Geometry check sheet. Reference: the model listing, model coordinates, mm. A direction names the side the tool comes from. Coordinates: 2 decimals unless noted, no trailing zeros. Write each loop counter-clockwise with the first axis right and the second up, starting at its lowest first coordinate (ties: lowest second). Pieces come first, ordered by that corner, then holes. Notation, with made-up numbers: M -8.5,70 L 33.5,70 A13 ccw 33.5,85 Z; hole C -23.5,2 d10. An arc over 180 degrees is marked long. Answer as a JSON object with one key per item and string values. Group by question number.
```python
from build123d import *

# Parameters (mm, degrees)
SKETCH_1_W               = 800
SKETCH_1_H               = 2000
EXTRUDE_1_DEPTH          = 50
SKETCH_2_W               = 20
SKETCH_2_H               = 100
EXTRUDE_2_DEPTH          = 50
SKETCH_3_R               = 20
EXTRUDE_3_DEPTH          = 100
PATTERN_LINEAR_1_COUNT   = 2
PATTERN_LINEAR_1_PITCH   = 1200
SKETCH_4_R               = 30
EXTRUDE_4_DEPTH          = 10
SKETCH_5_R               = 10
EXTRUDE_5_DEPTH          = 40
EXTRUDE_6_DEPTH          = 20
FILLET_1_R               = 10
MIRROR_START             = 610
MIRROR_1_DEPTH           = 120
MIRROR_2_COPY_1_SKETCH_W = 20
MIRROR_2_COPY_1_SKETCH_H = 100
MIRROR_2_COPY_1_DEPTH    = 50
MIRROR_2_COPY_2_SKETCH_R = 20
MIRROR_2_COPY_2_DEPTH    = 100
DELETE_START             = 405
DELETE_FACE_1_DEPTH      = 1300


with BuildPart() as part:
    # Эскиз1 → Бобышка-Вытянуть1 (new body)
    with BuildSketch(Plane(origin=(46095.73955041, 0, 0), x_dir=(-1, 0, 0), z_dir=(0, 0, -1))):
        with Locations((45695.73955041, 1000)):
            Rectangle(SKETCH_1_W, SKETCH_1_H)
    extrude(amount=-EXTRUDE_1_DEPTH)

    # Эскиз2 → Бобышка-Вытянуть2 (add)
    with BuildSketch(Plane(origin=(0, 0, 0), x_dir=(-1, 0, 0), z_dir=(0, 0, -1))):
        with Locations((-10, 1655)):
            Rectangle(SKETCH_2_W, SKETCH_2_H)
    extrude_2 = extrude(amount=EXTRUDE_2_DEPTH)

    # Эскиз3 → Бобышка-Вытянуть3 (add)
    with BuildSketch(Plane(origin=(0, 1605, 0), x_dir=(-1, 0, 0), z_dir=(0, -1, 0))):
        with Locations((5, 30)):
            Circle(SKETCH_3_R)
    extrude_3 = extrude(amount=-EXTRUDE_3_DEPTH)

    # Линейный массив1: Бобышка-Вытянуть2, Бобышка-Вытянуть3 ×2
    with Locations(*[(0, -i * PATTERN_LINEAR_1_PITCH, 0) for i in range(1, PATTERN_LINEAR_1_COUNT)]):
        add(extrude_2)
        add(extrude_3)

    # Эскиз4 → Бобышка-Вытянуть4 (add)
    with BuildSketch(Plane(origin=(0, 0, 0), x_dir=(-1, 0, 0), z_dir=(0, 0, -1))):
        with Locations((-730, 1000)):
            Circle(SKETCH_4_R)
    extrude(amount=EXTRUDE_4_DEPTH)

    # Эскиз5 → Бобышка-Вытянуть5 (add)
    with BuildSketch(Plane(origin=(0, 0, -10), x_dir=(-1, 0, 0), z_dir=(0, 0, -1))):
        with Locations((-730, 1000)):
            Circle(SKETCH_5_R)
    extrude(amount=EXTRUDE_5_DEPTH)

    # Эскиз6 → Бобышка-Вытянуть6 (add)
    with BuildSketch(Plane(origin=(0, 0, -50), x_dir=(-1, 0, 0), z_dir=(0, 0, -1))):
        with BuildLine():
            Line((-730, 1010), (-610, 1010))
            ThreePointArc((-610, 1010), (-600, 1000), (-610, 990))
            Line((-610, 990), (-730, 990))
            ThreePointArc((-730, 990), (-740, 1000), (-730, 1010))
        make_face()
    extrude(amount=EXTRUDE_6_DEPTH)

    # Скругление1
    # the kernel refuses this fillet: 10 mm, written as the material it takes off along each edge
    with BuildSketch(Plane(origin=(755, 1010, -50), x_dir=(0, -1, 0), z_dir=(-1, 0, 0))) as fillet_1_piece_1_section:
        with BuildLine():
            CenterArc((FILLET_1_R, -FILLET_1_R), FILLET_1_R, 90, 90)
            Line((0, -FILLET_1_R), (0, 0))
            Line((0, 0), (FILLET_1_R, 0))
        make_face()
    fillet_1_piece_1 = extrude(amount=145, mode=Mode.PRIVATE)
    fillet_1_piece_1 = fillet_1_piece_1 - Plane(origin=(730, 1000, -50), x_dir=(-1, 0, 0), z_dir=(0, 0, 1)) * Cylinder(10, 330, mode=Mode.PRIVATE)
    add(fillet_1_piece_1, mode=Mode.SUBTRACT)
    with BuildSketch(Plane(origin=(610, 1000, -50), x_dir=(0, 1, 0), z_dir=(1, 0, 0))) as fillet_1_piece_2:
        with BuildLine():
            CenterArc((10 - FILLET_1_R, -FILLET_1_R), FILLET_1_R, 0, 90)
            Line((10, -FILLET_1_R), (10, 0))
            Line((10, 0), (10 - FILLET_1_R, 0))
        make_face()
    revolve(axis=Axis((610, 1000, -50), (0, 0, 1)), revolution_arc=180, mode=Mode.SUBTRACT)
    with BuildSketch(Plane(origin=(730, 1010, -70), x_dir=(0, 0, 1), z_dir=(-1, 0, 0)), Plane(origin=(610, 990, -70), x_dir=(0, 0, 1), z_dir=(1, 0, 0))) as fillet_1_piece_3:
        with BuildLine():
            CenterArc((FILLET_1_R, -FILLET_1_R), FILLET_1_R, 90, 90)
            Line((0, -FILLET_1_R), (0, 0))
            Line((0, 0), (FILLET_1_R, 0))
        make_face()
    extrude(amount=120, mode=Mode.SUBTRACT)
    with BuildSketch(Plane(origin=(610, 1000, -70), x_dir=(0, 1, 0), z_dir=(1, 0, 0))) as fillet_1_piece_4:
        with BuildLine():
            CenterArc((10 - FILLET_1_R, FILLET_1_R), FILLET_1_R, 270, 90)
            Line((10 - FILLET_1_R, 0), (10, 0))
            Line((10, 0), (10, FILLET_1_R))
        make_face()
    revolve(axis=Axis((610, 1000, -70), (0, 0, 1)), revolution_arc=180, mode=Mode.SUBTRACT)
    with BuildSketch(Plane(origin=(730, 1000, -70), x_dir=(0, -1, 0), z_dir=(-1, 0, 0))) as fillet_1_piece_5:
        with BuildLine():
            CenterArc((10 - FILLET_1_R, FILLET_1_R), FILLET_1_R, 270, 90)
            Line((10 - FILLET_1_R, 0), (10, 0))
            Line((10, 0), (10, FILLET_1_R))
        make_face()
    revolve(axis=Axis((730, 1000, -70), (0, 0, 1)), revolution_arc=180, mode=Mode.SUBTRACT)
    with BuildSketch(Plane(origin=(730, 1000, -10), x_dir=(-1, 0, 0), z_dir=(0, -1, 0))) as fillet_1_piece_6:
        with BuildLine():
            CenterArc((30 - FILLET_1_R, -FILLET_1_R), FILLET_1_R, 0, 90)
            Line((30 - FILLET_1_R, 0), (30, 0))
            Line((30, 0), (30, -FILLET_1_R))
        make_face()
    revolve(axis=Axis((730, 1000, -10), (0, 0, -1)), mode=Mode.SUBTRACT)
    with BuildSketch(Plane(origin=(610, 990, -50), x_dir=(0, 1, 0), z_dir=(1, 0, 0))) as fillet_1_piece_7_section:
        with BuildLine():
            CenterArc((FILLET_1_R, -FILLET_1_R), FILLET_1_R, 90, 90)
            Line((0, -FILLET_1_R), (0, 0))
            Line((0, 0), (FILLET_1_R, 0))
        make_face()
    fillet_1_piece_7 = extrude(amount=145, mode=Mode.PRIVATE)
    fillet_1_piece_7 = fillet_1_piece_7 - Plane(origin=(730, 1000, -50), x_dir=(-1, 0, 0), z_dir=(0, 0, 1)) * Cylinder(10, 330, mode=Mode.PRIVATE)
    add(fillet_1_piece_7, mode=Mode.SUBTRACT)



with BuildPart() as body_2:
    # Зеркальное отражение1: read off the stored shape, not the designer's step
    # Зеркальное отражение1 outline → Зеркальное отражение1 (new body)
    with BuildSketch(Plane.YZ.offset(MIRROR_START)):
        with BuildLine():
            ThreePointArc((1000, 120), (992.928932188, 117.071067812), (990, 110))
            ThreePointArc((990, 110), (992.928932188, 102.928932188), (1000, 100))
            ThreePointArc((1000, 100), (1007.071067812, 102.928932188), (1010, 110))
            ThreePointArc((1010, 110), (1007.071067812, 117.071067812), (1000, 120))
        make_face()
    extrude(amount=MIRROR_1_DEPTH)


with BuildPart() as part_1:
    add(part.part)

    add(body_2.part)  # Mirror 1 2 merges body 2
    # Mirror 1 2 outline → Mirror 1 2 (revolve)
    with BuildSketch(Plane(origin=(730, 1000, 0), x_dir=(1, 0, 0), z_dir=(0, -1, 0))):
        with BuildLine():
            Line((10, 60), (10, 110))
            ThreePointArc((10, 110), (7.071067812, 117.071067812), (0, 120))
            Line((0, 120), (0, 50))
            Line((0, 50), (30, 50))
            ThreePointArc((30, 50), (27.071067812, 57.071067812), (20, 60))
            Line((20, 60), (10, 60))
        make_face()
    revolve(axis=Axis((730, 1000, 0), (0, 0, 1)))

    # Mirror 1 3 outline → Mirror 1 3 (revolve)
    with BuildSketch(Plane(origin=(0, 1000, 110), x_dir=(0, 1, 0), z_dir=(0, 0, -1))):
        with BuildLine():
            Line((0, 610), (0, 600))
            ThreePointArc((0, 600), (7.071067812, 602.928932188), (10, 610))
            Line((10, 610), (0, 610))
        make_face()
    revolve(axis=Axis((0, 1000, 110), (1, 0, 0)))

    # Зеркальное отражение2: Бобышка-Вытянуть2, Бобышка-Вытянуть3 across plane
    add(extrude_2.mirror(Plane(origin=(0, 0, 25), x_dir=(1, 0, 0), z_dir=(0, 0, -1))))
    add(extrude_3.mirror(Plane(origin=(0, 0, 25), x_dir=(1, 0, 0), z_dir=(0, 0, -1))))

    # Зеркальное отражение2 copy 1 sketch → Зеркальное отражение2 copy 1 (add)
    with BuildSketch(Plane(origin=(0, -1200, 50), x_dir=(-1, 0, 0), z_dir=(0, 0, 1))):
        with Locations((-10, -1655)):
            Rectangle(MIRROR_2_COPY_1_SKETCH_W, MIRROR_2_COPY_1_SKETCH_H)
    extrude(amount=MIRROR_2_COPY_1_DEPTH)

    # Зеркальное отражение2 copy 2 sketch → Зеркальное отражение2 copy 2 (add)
    with BuildSketch(Plane(origin=(0, 405, 50), x_dir=(-1, 0, 0), z_dir=(0, -1, 0))):
        with Locations((5, -30)):
            Circle(MIRROR_2_COPY_2_SKETCH_R)
    extrude(amount=-MIRROR_2_COPY_2_DEPTH)

    # Delete Face 1: read off the stored shape, not the designer's step
    # Delete Face 1 outline → Delete Face 1 (cut)
    with BuildSketch(Plane(origin=(0, 0, 0), x_dir=(1, 0, 0), z_dir=(0, 1, 0)).offset(DELETE_START)):
        with BuildLine():
            Line((20, 50), (0, 50))
            Line((0, 50), (0, 49.364916731))
            ThreePointArc((0, 49.364916731), (-25, 30), (0, 10.635083269))
            Line((0, 10.635083269), (0, 0))
            Line((0, 0), (20, 0))
            Line((20, 0), (20, 50))
        make_face()
    extrude(amount=DELETE_FACE_1_DEPTH, mode=Mode.SUBTRACT)


solid = part_1.part
```
1) Go/stop test with flat-tipped pins: pin 1 Ø12 at (x, y) = (584, 748) entering from -Z; pin 2 Ø3 at (x, y) = (607, 836.5) entering from +Z; pin 3 Ø25 at (y, z) = (451, 66.5) entering from +X. Record where each tip stops, or that it passes through.
2) Set-up check for faces 4 (the flat face through (721, 1005, 60)), 5 (the flat face through (3, 505, 75)), 6 (the flat face through (3, 405, 75)): record each of +Z, -Z, +X, -X, +Y, -Y from which the full face is reachable in a straight line by a thin tool's end or side.
3) Section check A-A (z = 80). Record the cut outline in (x, y), then the cut area to 3 significant figures.
4) Material ranges on probe 1 along Z at (x, y) = (727, 625); probe 2 along X at (y, z) = (1743.5, 10); probe 3 along Y at (x, z) = (732, 86.5), recorded low to high. Write a range as [from, to].
5) Section check C-C (y = 1371). Record the cut outline in (x, z).
6) Section check B-B (x = 133.5). Record the cut outline in (y, z).
7) Draft check along Y on faces 1 (the flat face through (3, 1605, 75)), 2 (the flat face through (406, 0, 25)), 3 (the flat face through (20, 1654, 75)). Enter one of: +Y half, -Y half, draft (parallel to the pull), parting line (faces both ways), or undercut.
Entries:
{
 "1": {"pin 1": "z = 0", "pin 2": "z = 50", "pin 3": "x = 20"},
 "2": {"face 4": "none", "face 5": "+Z, +X, -X", "face 6": "+Z, +X, -X, -Y"},
 "3": {"outline": "M -25,405 L 20,405 L 20,505 L -25,505 Z; M -25,1605 L 20,1605 L 20,1705 L -25,1705 Z; C 730,1000 d20", "area": "9,310 mm^2"},
 "4": {"probe 1": "[0, 50]", "probe 2": "[0, 800]", "probe 3": "[990.2, 1009.8]"},
 "5": {"outline": "M 0,0 L 800,0 L 800,50 L 0,50 Z"},
 "6": {"outline": "M 0,0 L 2000,0 L 2000,50 L 0,50 Z"},
 "7": {"face 1": "undercut", "face 2": "-Y half", "face 3": "draft"}
}
